Autodesk Inventor part; units mm, degrees
ref_plane "YZ Plane" through (0, 0, 0) normal (1, 0, 0) x (0, 1, 0)
ref_plane "XZ Plane" through (0, 0, 0) normal (0, 1, 0) x (-1, 0, 0)
ref_plane "XY Plane" through (0, 0, 0) normal (0, 0, 1) x (1, 0, 0)
sketch "Skizze1" plane through (0, 0, 0) normal (0, 0, 1) x (1, 0, 0)
  line L0 (5, 5) -> (5, 50)
  line L1 (5, 50) -> (0, 50)
  line L2 (0, 50) -> (0, 0)
  line L3 (5, 5) -> (50, 5)
  line L4 (50, 5) -> (50, 0)
  line L5 (-10, 0) -> (60, 0)
  line L6 (0, -10) -> (0, 60)
  line L7 (0, 0) -> (50, 0)
  dimension "d3" = 5
  dimension "d4" = 5
  dimension "d5" = 50
  dimension "d6" = 50
extrude "Extrusion1" add sketch "Skizze1" along normal blind 25
sketch "Skizze2" plane through (0, 0, 0) normal (0, -1, 0) x (1, 0, 0)
  line L0 (0, 0) -> (0, 25)
  line L1 (50, 0) -> (50, 25)
  line L2 (5, 0) -> (5, 25)
  line L3 (5, 20.5) -> (36, 20.5)
  line L4 (36, 20.5) -> (36, 4.5)
  line L5 (36, 4.5) -> (5, 4.5)
  line L6 (0, 12.5) -> (50, 12.5)
  line L7 (5, 25) -> (50, 25)
  line L8 (50, 25) -> (50, 0)
  line L9 (50, 0) -> (5, 0)
  line L10 (5, 0) -> (5, 4.5)
  line L11 (5, 20.5) -> (5, 25)
  dimension "d9" = 16
  dimension "d11" = 36
extrude "Extrusion2" cut sketch "Skizze2" against normal through all contours L9 L2 L5 L4 L6 L1 | L6 L4 L3 L2 L7 L1
sketch "Skizze3" plane through (0, 0, 0) normal (0, -1, 0) x (1, 0, 0)
  line L0 (5, 4.5) -> (36, 4.5)
  line L1 (36, 4.5) -> (36, 20.5)
  line L2 (36, 20.5) -> (5, 20.5)
  line L3 (0, 0) -> (0, 25)
  line L4 (36, 12.5) -> (0, 12.5)
  line L5 (20.5, 20.5) -> (20.5, 4.5)
  point P0 (20.5, 12.5)
hole "Bohrung1" at (20.5, 0, 12.5) direction (0, 1, 0) diameter 4.1 end through all
sketch "Skizze4" plane through (0, 0, 0) normal (0, -1, 0) x (1, 0, 0)
  line L0 (5, 4.5) -> (36, 4.5)
  line L1 (36, 4.5) -> (36, 20.5)
  line L2 (36, 20.5) -> (5, 20.5)
  line L3 (0, 0) -> (0, 25)
  line L4 (20.5, 20.5) -> (20.5, 4.5)
  line L5 (0, 12.5) -> (36, 12.5)
  point P0 (11.5, 12.5)
  point P1 (29.5, 12.5)
  dimension "d21" = 18
hole "Bohrung2" at (11.5, 0, 12.5) at (29.5, 0, 12.5) direction (0, 1, 0) diameter 3.4 end through all
fillet "Rundung1" radius 4 2 edges at (5, 2.5, 20.5) (5, 2.5, 4.5)
sketch "Skizze5" plane through (5, 0, 0) normal (1, 0, 0) x (0, 0, -1)
  line L0 (0, 50) -> (-25, 50)
  line L1 (-0.5, 5) -> (-24.5, 5)
  line L2 (-12.5, 50) -> (-12.5, 9.3168)
  point P0 (-12.5, 40)
  point P1 (-12.5, 22)
  dimension "d30" = 10
  dimension "d31" = 18
hole "Bohrung3" at (5, 40, 12.5) at (5, 22, 12.5) direction (-1, 0, 0) diameter 4.5 end through all countersink diameter 9.2 countersink angle 90
properties part number "1_0204_013"
Geometry check sheet. Reference: the model listing, model coordinates, mm. A direction names the side the tool comes from. Round coordinates to 2 decimals unless told otherwise and drop trailing zeros. Loops run counter-clockwise (first coordinate to the right, second up) from the corner with the lowest first, then second, coordinate; pieces in that order, holes last. Notation, with made-up numbers: M 84.25,13 L 132.25,13 A23 cw 132.25,34 Z; hole C 42.5,-19.5 d10. An arc over 180 degrees is marked long. Return JSON: item names as keys, results as strings. Group by question number.
(1) Section check C-C, the plane y = 22. Enter the section's corners in (x, z), and give its area (3 significant figures).
(2) Section check B-B, the plane z = 12.5. Give the number of separate pieces and of enclosed holes in the cut face, and give its area (3 significant figures).
(3) Set-up check for faces 1 (the face through (2, 25, 0)), 2 (the face through (23, 2, 4.5)): record each of +Z, -Z, +X, -X, +Y, -Y from which the full face is reachable in a straight line by a thin tool's end or side.
(4) Scan lines: line 1 along X through (y, z) = (2.55, 12.5); line 2 along Z through (x, y) = (20.5, 3.7); line 3 along Z through (x, y) = (1, 40). Record each from-to range of solid material in increasing order. Write a range as [from, to].
(5) Go/stop test with flat-tipped pins: pin 1 (1 mm diameter, centred on x = 11.5, z = 18, fed in from +Y); pin 2 (4 mm diameter, centred on x = 23, y = 3.5, fed in from +Z); pin 3 (5 mm diameter, centred on y = 12.5, z = 8, fed in from +X); pin 4 (3.5 mm diameter, centred on x = 20.5, z = 12.5, fed in from -Y). Record where each tip stops, or that it passes through.
(6) Mould release check, pull along X, two halves, no side actions. Record for faces 3 (the face through (0, 25, 12)), 4 (the face through (36, 2, 13)), 5 (the face through (22, 2, 20.5)), 6 (the face through (13, 2.5, 11.7)): pulls with the +X half, pulls with the -X half, needs draft (parallel to the pull), parting line crosses it, or undercut.
(7) Section check A-A, the plane x = 20.5. Enter the section's corners in (y, z).
(8) Section check D-D, the plane x = 29.5. Enter the section's corners in (y, z), and give its area (3 significant figures).
Data:
{
 "1": {"outline": "M 0,0 L 5,0 L 5,7.9 L 2.65,10.25 L 0,10.25 Z; M 0,14.75 L 2.65,14.75 L 5,17.1 L 5,25 L 0,25 Z", "area": "97.0 mm²"},
 "2": {"separate pieces": "6", "enclosed holes": "0", "area": "294 mm²"},
 "3": {"face 1": "-Z, +X, -X, +Y, -Y", "face 2": "-Z, +X, +Y, -Y"},
 "4": {"line 1": "[0, 9.8], [13.2, 18.45], [22.55, 27.8], [31.2, 36]", "line 2": "[4.5, 10.45], [14.55, 20.5]", "line 3": "[0, 10.25], [14.75, 25]"},
 "5": {"pin 1": "y = 5", "pin 2": "z = 20.5", "pin 3": "x = 5", "pin 4": "through"},
 "6": {"face 3": "pulls with the -X half", "face 4": "pulls with the +X half", "face 5": "needs draft", "face 6": "undercut"},
 "7": {"outline": "M 0,4.5 L 5,4.5 L 5,10.45 L 0,10.45 Z; M 0,14.55 L 5,14.55 L 5,20.5 L 0,20.5 Z"},
 "8": {"outline": "M 0,4.5 L 5,4.5 L 5,10.8 L 0,10.8 Z; M 0,14.2 L 5,14.2 L 5,20.5 L 0,20.5 Z", "area": "63.0 mm²"}
}
